from build123d import *

# Parameters (mm, degrees)
SKETCH_W                   = 55.5
SKETCH_H                   = 55.5
PAD_DEPTH                  = 2
SKETCH001_R                = 2
POCKET_DEPTH               = 159.02966
SKETCH002_R                = 4
POCKET001_DEPTH            = 1
SKETCH001_MIRRORED_2_R     = 2
POCKET_MIRRORED_2_DEPTH    = 159.02966
SKETCH002_MIRRORED_2_R     = 4
POCKET001_MIRRORED_2_DEPTH = 1
FILLET_R                   = 3
FILLET001_R                = 1.5


with BuildPart() as part:
    # Sketch → Pad (new body)
    with BuildSketch(Plane.XY):
        Rectangle(SKETCH_W, SKETCH_H)
    extrude(amount=PAD_DEPTH)

    # Sketch001 (on Face6 of Pad) → Pocket (cut, through all)
    with BuildSketch(Plane.XY.offset(2)):
        with Locations((21.25, 21.25)):
            Circle(SKETCH001_R)
    pocket = extrude(amount=-POCKET_DEPTH, mode=Mode.SUBTRACT)

    # Sketch002 (on Face5 of Pocket) → Pocket001 (cut)
    with BuildSketch(Plane.XY.offset(2)):
        with Locations((21.25, 21.25)):
            Circle(SKETCH002_R)
    pocket001 = extrude(amount=-POCKET001_DEPTH, mode=Mode.SUBTRACT)

    # Sketch001 Mirrored 2 → Pocket Mirrored 2 (cut, through all)
    with BuildSketch(Plane(origin=(0, 0, 2), x_dir=(-1, 0, 0), z_dir=(0, 0, -1))):
        with Locations((21.25, 21.25)):
            Circle(SKETCH001_MIRRORED_2_R)
    pocket_mirrored_2 = extrude(amount=POCKET_MIRRORED_2_DEPTH, mode=Mode.SUBTRACT)

    # Sketch002 Mirrored 2 → Pocket001 Mirrored 2 (cut)
    with BuildSketch(Plane(origin=(0, 0, 2), x_dir=(-1, 0, 0), z_dir=(0, 0, -1))):
        with Locations((21.25, 21.25)):
            Circle(SKETCH002_MIRRORED_2_R)
    pocket001_mirrored_2 = extrude(amount=POCKET001_MIRRORED_2_DEPTH, mode=Mode.SUBTRACT)

    # Mirrored001: Pocket, Pocket001, Pocket Mirrored 2, Pocket001 Mirrored 2 across Sketch001 H_Axis
    add(pocket.mirror(Plane(origin=(0, 0, 2), x_dir=(0, 0, 1), z_dir=(0, 1, 0))), mode=Mode.SUBTRACT)
    add(pocket001.mirror(Plane(origin=(0, 0, 2), x_dir=(0, 0, 1), z_dir=(0, 1, 0))), mode=Mode.SUBTRACT)
    add(pocket_mirrored_2.mirror(Plane(origin=(0, 0, 2), x_dir=(0, 0, 1), z_dir=(0, 1, 0))), mode=Mode.SUBTRACT)
    add(pocket001_mirrored_2.mirror(Plane(origin=(0, 0, 2), x_dir=(0, 0, 1), z_dir=(0, 1, 0))), mode=Mode.SUBTRACT)

    # Fillet
    fillet_edges = [part.edges().sort_by_distance(p)[0] for p in [
        (-27.75, -27.75, 1),
        (27.75, -27.75, 1),
        (27.75, 27.75, 1),
        (-27.75, 27.75, 1),
    ]]
    fillet(fillet_edges, radius=FILLET_R)

    # Fillet001
    fillet001_edges = [part.edges().sort_by_distance(p)[0] for p in [
        (0, -27.75, 2),
    ]]
    fillet(fillet001_edges, radius=FILLET001_R)


solid = part.part
The model under review builds one solid part; all positions refer to its coordinate system, in mm. A direction names the side the tool comes from. Coordinates: 2 decimals unless noted, no trailing zeros. Loops run counter-clockwise (first coordinate to the right, second up) from the corner with the lowest first, then second, coordinate; pieces in that order, holes last.
(1) Wall thickness on L1, parallel to Y at x = 21.25, z = 0.75; L2, parallel to Y at x = 22, z = 0.4; L3, parallel to X at y = -21.25, z = 1.65: over which ranges is each line inside the solid? List them lowest first.
Determined:
L1: y = -27.73 to -23.25, -19.25 to 19.25, 23.25 to 27.73
L2: y = -27.75 to -23.1, -19.4 to 19.4, 23.1 to 27.75
L3: x = -27.21 to -25.25, -17.25 to 17.25, 25.25 to 27.21
(2) Draft analysis for pull direction Y (two halves, no side actions). For faces 3 (the cylindrical face through (26.85, -26.89, 0.25)), 4 (the cylindrical face through (-0.35, 27.3, 1.57)), 5 (the flat face through (-19, 20, 1)), 6 (the cylindrical face through (20.729, 25.216, 1.507)), state which applies: +Y half, -Y half, draft (parallel to the pull), parting line (faces both ways), or undercut.
Determined:
face 3: -Y half
face 4: +Y half
face 5: undercut
face 6: undercut
(3) Insertion check: P1, Ø2.5, axis at x = -21.5, y = -22, coming from the +Z side; P2, Ø2.5, axis at x = 21.25, y = 21.25, coming from the -Z side. Each pin has a flat end and moves straight along its axis. Give the tip position at first contact, or say it passes through.
Determined:
P1: stops at z = 1
P2: passes through
(4) Consider section A-A, the plane x = 21.25. Give the boundary of the cut face in (y, z), plus the area to 3 significant figures.
Determined:
outline: (-27.75, 0) - (-23.25, 0) - (-23.25, 1) - (-25.25, 1) - (-25.25, 2) - (-26.25, 2) arc R1.5 ccw to (-27.75, 0.5) - close; (-19.25, 0) - (19.25, 0) - (19.25, 1) - (17.25, 1) - (17.25, 2) - (-17.25, 2) - (-17.25, 1) - (-19.25, 1) - close; (23.25, 0) - (27.75, 0) - (27.75, 0.5) arc R1.5 ccw to (26.25, 2) - (25.25, 2) - (25.25, 1) - (23.25, 1) - close
area: 86.0 mm2
(5) Tool access review of faces 1 (the cylindrical face through (20.729, -25.216, 1.507)), 2 (the flat face through (0, 0, 0)): name each direction out of +Z, -Z, +X, -X, +Y, -Y from which nothing blocks a thin tool from reaching the whole face with its end or side.
Determined:
face 1: +Z
face 2: -Z, +X, -X, +Y, -Y
(6) Consider section C-C, the plane z = 1.6. Give the number of separate pieces and of enclosed holes in the cut face, plus the area to 3 significant figures.
Determined:
separate pieces: 1
enclosed holes: 4
area: 2,770 mm2
